Model file for the job. Use its own axes, mm. Face numbers are marked on the shaded views. A direction names the side the tool comes from. Round coordinates to 2 decimals unless told otherwise and drop trailing zeros. Order: outer loops, then holes, each group sorted by start corner. A loop starts at its lowest first (then second) coordinate and runs counter-clockwise, first axis right, second up. Notation, with made-up numbers: (-23, 68) -> (14, 68) arc R21 cw to (14, 98) -> close; hole circle Ø8 at (87.25, 62.5). An arc over 180 degrees is marked (long way). Put each result on its own line as item: value. Start each with the question number.
Q1. Flat gauge pins, fed straight in: P1, Ø10, axis at y = 82, z = 2.5, coming from the +X side; P2, Ø1.5, axis at y = 31.5, z = -11, coming from the +X side; P3, Ø2, axis at y = 51.5, z = -17, coming from the -X side. Where does each tip first touch, or does it go through?
Q2. Cut at A-A, the plane x = 0. List the corners of the cut face in (y, z), and give its area (3 significant figures).
Q3. Cut at C-C, the plane y = 49.5. List the corners of the cut face in (x, z), and give its area (3 significant figures).
Q4. Probe L1, parallel to Z at x = 1, y = 35.5; L2, parallel to X at y = 16.5, z = 9.5; L3, parallel to X at y = 59, z = 18.5. List the from-to ranges inside material, lowest first.
Q5. Cut at B-B, the plane z = 0. List the corners of the cut face in (x, y), and give its area (3 significant figures).
Q6. 3-axis set-ups, long thin cutter, end or side, ignore diameter. For the marked faces 1 and 2: which of +Z, -Z, +X, -X, +Y, -Y reach the whole face in a straight line?
Autodesk Inventor part; units mm, degrees
ref_plane "YZ Plane" through (0, 0, 0) normal (1, 0, 0) x (0, 1, 0)
ref_plane "XZ Plane" through (0, 0, 0) normal (0, 1, 0) x (-1, 0, 0)
ref_plane "XY Plane" through (0, 0, 0) normal (0, 0, 1) x (1, 0, 0)
sketch "Sketch1" plane through (0, 0, 0) normal (0, 1, 0) x (-1, 0, 0)
  circle A0 centre (0, 0) radius 23.5
  dimension "d0" = 47
extrude "Extrusion1" add sketch "Sketch1" along normal blind 80
sketch "Sketch2" plane through (0, 80, 0) normal (0, 1, 0) x (1, 0, 0)
  circle A0 centre (0, 0) radius 17.5
  dimension "d3" = 35
extrude "Extrusion2" add sketch "Sketch2" along normal blind 5
sketch "Sketch3" plane through (0, 85, 0) normal (0, 1, 0) x (1, 0, 0)
  circle A0 centre (0, 0) radius 20
  dimension "d6" = 40
extrude "Extrusion3" add sketch "Sketch3" along normal blind 10
fillet "Fillet1" radius 2 1 edges at (23.5, 0, 0)
fillet "Fillet2" radius 5 1 edges at (23.5, 80, 0)
properties part number "Tarro"
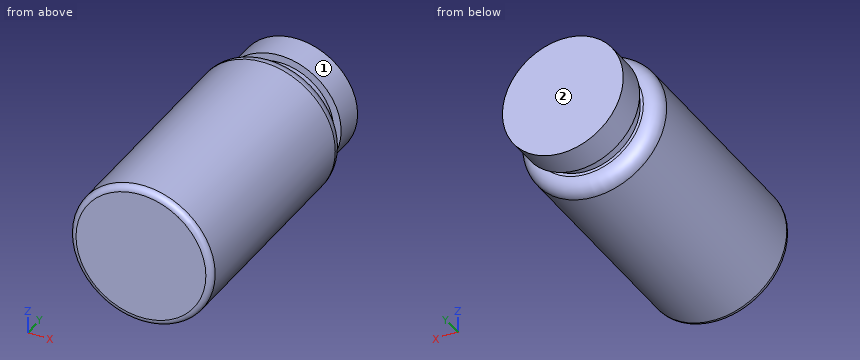
Ans:
1. P1: stops at x = 22.99
1. P2: stops at x = 21.15
1. P3: stops at x = -17.21
2. outline: (0, -21.5) arc R2 ccw to (2, -23.5) -> (75, -23.5) arc R5 ccw to (80, -18.5) -> (80, -17.5) -> (85, -17.5) -> (85, -20) -> (95, -20) -> (95, 20) -> (85, 20) -> (85, 17.5) -> (80, 17.5) -> (80, 18.5) arc R5 ccw to (75, 23.5) -> (2, 23.5) arc R2 ccw to (0, 21.5) -> close
2. area: 4,320 mm^2
3. outline: circle Ø47 at (0, 0)
3. area: 1,730 mm^2
4. L1: z = -23.48 to 23.48
4. L2: x = -21.49 to 21.49
4. L3: x = -14.49 to 14.49
5. outline: (-23.5, 2) arc R2 ccw to (-21.5, 0) -> (21.5, 0) arc R2 ccw to (23.5, 2) -> (23.5, 75) arc R5 ccw to (18.5, 80) -> (17.5, 80) -> (17.5, 85) -> (20, 85) -> (20, 95) -> (-20, 95) -> (-20, 85) -> (-17.5, 85) -> (-17.5, 80) -> (-18.5, 80) arc R5 ccw to (-23.5, 75) -> close
5. area: 4,320 mm^2
6. face 1: +Y
6. face 2: +Z, -Z, +X, -X, +Y
